Verification items for the finished model (mm, model axes). Face numbers are marked on the shaded views. Coordinates: 2 decimals unless noted, no trailing zeros. Order: outer loops, then holes, each group sorted by start corner. A loop starts at its lowest first (then second) coordinate and runs counter-clockwise, first axis right, second up. Notation, with made-up numbers: M 2,30 L 49,30 A9 ccw 49,44 Z; hole C -26,-8 d5. An arc over 180 degrees is marked long. Return JSON: item names as keys, results as strings. Group by question number.
1. Section check B-B, the plane x = 39.5. Record the cut outline in (y, z), plus the area to 3 significant figures.
2. Material ranges on line 1 along Z through (x, y) = (10.5, 1.4); line 2 along X through (y, z) = (2.4, -17.5); line 3 along X through (y, z) = (1.9, -18), recorded low to high.
3. Section check A-A, the plane y = 4.55. Give the number of separate pieces and of enclosed holes in the cut face, plus the area to 3 significant figures.
4. Mould release check, pull along X, two halves, no side actions. Record for the marked faces 1, 2, 3 and 4: +X half, -X half, draft (parallel to the pull), parting line (faces both ways), or undercut.
5. Gauge pin test, flat ends, axial feed: pin 1 (1.5 mm diameter, centred on x = -19.5, z = 14.5, fed in from -Y); pin 2 (2 mm diameter, centred on x = -10, y = 3, fed in from +Z); pin 3 (1 mm diameter, centred on y = 1, z = 10, fed in from -X). Record the tip position at first contact, or that the pin passes through.
```python
from build123d import *

# Parameters (mm, degrees)
SKETCH1_R           = 1
BOSS_EXTRUDE1_DEPTH = 6
FILLET1_R           = 7.5


with BuildPart() as part:
    # Sketch1 → Boss-Extrude1 (new body)
    with BuildSketch(Plane(origin=(0, 0, 0), x_dir=(1, 0, 0), z_dir=(0, 1, 0))):
        with BuildLine():
            Line((31.883633055, 20.164562188), (44.561021943, 28.182280752))
            ThreePointArc((44.561021943, 28.182280752), (52.725, 0), (44.561021943, -28.182280752))
            Line((44.561021943, -28.182280752), (31.883633055, -20.164562188))
            ThreePointArc((31.883633055, -20.164562188), (0, -37.725), (-31.883633055, -20.164562188))
            Line((-31.883633055, -20.164562188), (-44.561021943, -28.182280752))
            ThreePointArc((-44.561021943, -28.182280752), (-52.725, 0), (-44.561021943, 28.182280752))
            Line((-44.561021943, 28.182280752), (-31.883633055, 20.164562188))
            ThreePointArc((-31.883633055, 20.164562188), (0, 37.725), (31.883633055, 20.164562188))
        make_face()
        with Locations(Location((-11.083898795, 11.083898795, 0), (0, 0, 270))):
            Circle(SKETCH1_R, mode=Mode.SUBTRACT)
        with Locations(Location((11.083898795, 11.083898795, 0), (0, 0, 270))):
            Circle(SKETCH1_R, mode=Mode.SUBTRACT)
        with Locations(Location((11.083898795, -11.083898795, 0), (0, 0, 270))):
            Circle(SKETCH1_R, mode=Mode.SUBTRACT)
        with Locations(Location((-11.083898795, -11.083898795, 0), (0, 0, 270))):
            Circle(SKETCH1_R, mode=Mode.SUBTRACT)
        with Locations(Location((41.701925915, 17.5, 0), (0, 0, 270))):
            Circle(SKETCH1_R, mode=Mode.SUBTRACT)
        with Locations(Location((41.701925915, -17.5, 0), (0, 0, 270))):
            Circle(SKETCH1_R, mode=Mode.SUBTRACT)
        with Locations(Location((-41.701925915, 17.5, 0), (0, 0, 90))):
            Circle(SKETCH1_R, mode=Mode.SUBTRACT)
        with Locations(Location((-41.701925915, -17.5, 0), (0, 0, 90))):
            Circle(SKETCH1_R, mode=Mode.SUBTRACT)
    extrude(amount=BOSS_EXTRUDE1_DEPTH)

    # Fillet1
    fillet1_edges = [part.edges().sort_by_distance(p)[0] for p in [
        (44.561021943, 3, 28.182280752),
        (31.883633055, 3, 20.164562188),
        (-44.561021943, 3, 28.182280752),
        (-31.883633055, 3, 20.164562188),
        (44.561021943, 3, -28.182280752),
        (31.883633055, 3, -20.164562188),
        (-44.561021943, 3, -28.182280752),
        (-31.883633055, 3, -20.164562188),
    ]]
    fillet(fillet1_edges, radius=FILLET1_R - 0.0001)  # a hair under: the kernel refuses the full size


solid = part.part
```
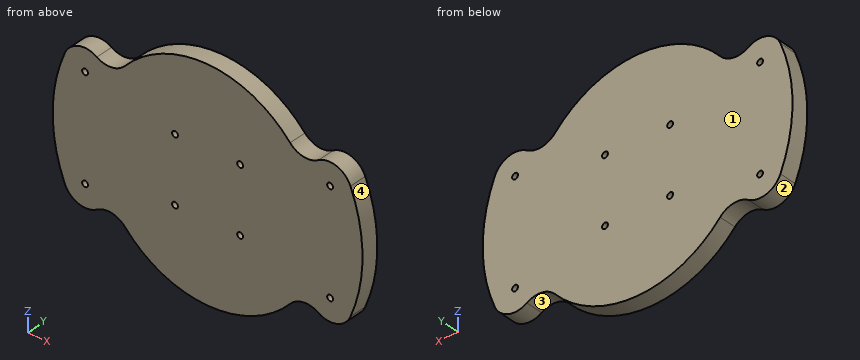
Answers follow:
{
 "1": {"outline": "M 0,-24.67 L 6,-24.67 L 6,24.67 L 0,24.67 Z", "area": "296 mm^2"},
 "2": {"line 1": "-36.23 to -11.9, -10.27 to 10.27, 11.9 to 36.23", "line 2": "-49.74 to -42.7, -40.7 to 40.7, 42.7 to 49.74", "line 3": "-49.56 to -42.57, -40.84 to 40.84, 42.57 to 49.56"},
 "3": {"separate pieces": "1", "enclosed holes": "8", "area": "5,950 mm^2"},
 "4": {"face 1": "draft", "face 2": "undercut", "face 3": "undercut", "face 4": "+X half"},
 "5": {"pin 1": "y = 0", "pin 2": "z = 36.64", "pin 3": "x = -51.86"}
}
